from build123d import *

# Parameters (mm, degrees)
BOSS_EXTRUDE1_DEPTH = 1.6
FILLET1_R           = 5
SKETCH2_R           = 1.25
SKETCH2_W           = 17
SKETCH2_H           = 6.4
SKETCH2_W_2         = 30
SKETCH2_H_2         = 8
CUT_EXTRUDE1_DEPTH  = 3
FILLET2_R           = 2


with BuildPart() as part:
    # Sketch1 → Boss-Extrude1 (new body)
    with BuildSketch(Plane(origin=(0, 0, 0), x_dir=(1, 0, 0), z_dir=(0, 1, 0))):
        Polygon((-20, 55.916666667), (20, 55.916666667), (35, 30.916666667), (35, 25.916666667), (25, 25.916666667), (25, -22.083333333), (-25, -22.083333333), (-25, 25.916666667), (-35, 25.916666667), (-35, 30.916666667), align=None)
    extrude(amount=BOSS_EXTRUDE1_DEPTH)

    # Fillet1
    # the kernel refuses this fillet: 5 mm, written as the material it takes off along each edge
    with BuildSketch(Plane(origin=(-20, -7.077379737, -55.916666667), x_dir=(1, 0, 0), z_dir=(0, 1, 0))) as fillet1_piece_1:
        with BuildLine():
            CenterArc((FILLET1_R * 0.566190378969, -FILLET1_R), FILLET1_R, 90, 59.036243468)
            Line((-FILLET1_R * 0.291302546743, -FILLET1_R * 0.485504244572), (0, 0))
            Line((0, 0), (FILLET1_R * 0.566190378969, 0))
        make_face()
    extrude(amount=15.754759474, mode=Mode.SUBTRACT)
    with BuildSketch(Plane(origin=(20, -7.077379737, -55.916666667), x_dir=(-1, 0, 0), z_dir=(0, 1, 0))) as fillet1_piece_2:
        with BuildLine():
            CenterArc((FILLET1_R * 0.566190378969, FILLET1_R), FILLET1_R, 210.963756532, 59.036243468)
            Line((-FILLET1_R * 0.291302546743, FILLET1_R * 0.485504244572), (0, 0))
            Line((0, 0), (FILLET1_R * 0.566190378969, 0))
        make_face()
    extrude(amount=15.754759474, mode=Mode.SUBTRACT)
    with BuildSketch(Plane(origin=(-35, -3.462299562, -30.916666667), x_dir=(0, 0, 1), z_dir=(0, 1, 0)), Plane(origin=(35, -3.462299562, -30.916666667), x_dir=(-0.5144957554275258, 0, -0.8574929257125447), z_dir=(0, 1, 0))) as fillet1_piece_3:
        with BuildLine():
            CenterArc((FILLET1_R * 0.276983964948, FILLET1_R), FILLET1_R, 239.036243468, 30.963756532)
            Line((-FILLET1_R * 0.237511790479, FILLET1_R * 0.142507074287), (0, 0))
            Line((0, 0), (FILLET1_R * 0.276983964948, 0))
        make_face()
    extrude(amount=8.524599124, mode=Mode.SUBTRACT)
    with BuildSketch(Plane(origin=(-25, -12.5, 22.083333333), x_dir=(1, 0, 0), z_dir=(0, 1, 0)), Plane(origin=(25, -12.5, 22.083333333), x_dir=(0, 0, -1), z_dir=(0, 1, 0)), Plane(origin=(-35, -12.5, -25.916666667), x_dir=(1, 0, 0), z_dir=(0, 1, 0)), Plane(origin=(35, -12.5, -25.916666667), x_dir=(0, 0, -1), z_dir=(0, 1, 0))) as fillet1_piece_4:
        with BuildLine():
            CenterArc((FILLET1_R, FILLET1_R), FILLET1_R, 180, 90)
            Line((0, FILLET1_R), (0, 0))
            Line((0, 0), (FILLET1_R, 0))
        make_face()
    extrude(amount=26.6, mode=Mode.SUBTRACT)

    # Sketch2 → Cut-Extrude1 (cut)
    with BuildSketch(Plane(origin=(0, 0, 0), x_dir=(1, 0, 0), z_dir=(0, 1, 0))):
        with Locations(Location((22.5, -17.083333333, 0), (0, 0, 90))):
            Circle(SKETCH2_R)
        with Locations(Location((21.5, -4.403333333, 0), (0, 0, 90))):
            Circle(SKETCH2_R)
        with Locations(Location((17.9, 31.906666667, 0), (0, 0, 90))):
            Circle(SKETCH2_R)
        with Locations(Location((21.5, 12.226666667, 0), (0, 0, 90))):
            Circle(SKETCH2_R)
        with Locations(Location((-17.9, 31.906666667, 0), (0, 0, 90))):
            Circle(SKETCH2_R)
        with Locations(Location((-21.5, 12.226666667, 0), (0, 0, 90))):
            Circle(SKETCH2_R)
        with Locations(Location((-21.5, -4.403333333, 0), (0, 0, 90))):
            Circle(SKETCH2_R)
        with Locations(Location((-22.5, -17.083333333, 0), (0, 0, 90))):
            Circle(SKETCH2_R)
        with Locations((16.5, 3.896666667)):
            Rectangle(SKETCH2_W, SKETCH2_H)
        with Locations((-16.5, 3.896666667)):
            Rectangle(SKETCH2_W, SKETCH2_H)
        with Locations((0, 46.916666667)):
            Rectangle(SKETCH2_W_2, SKETCH2_H_2)
    extrude(amount=CUT_EXTRUDE1_DEPTH, mode=Mode.SUBTRACT)

    # Fillet2
    fillet2_edges = [part.edges().sort_by_distance(p)[0] for p in [
        (8, 0.8, -7.096666667),
        (8, 0.8, -0.696666667),
        (-8, 0.8, -0.696666667),
        (-8, 0.8, -7.096666667),
    ]]
    fillet(fillet2_edges, radius=FILLET2_R)


solid = part.part
Work out the finished part from the listing and answer in its coordinate system (mm). A direction names the side the tool comes from. Give positions to 0.01 mm unless a question says otherwise; leave off trailing zeros. Loops run counter-clockwise (first coordinate to the right, second up) from the corner with the lowest first, then second, coordinate; pieces in that order, holes last. Notation, with made-up numbers: (15.25, -1) - (23.25, -1) arc R21 ccw to (23.25, 31) - close; hole circle Ø6 at (85.5, 41). An arc over 180 degrees is marked (long way). Answer in a Markdown table with one row per item. Add a question column.
Q1. A tool of negligible diameter and unlimited length cuts with its end or side. For faces 1 (the cylindrical face through (8.57, 0.811, -6.495)), 2 (the flat face through (-18, 1, -0.697)), 3 (the flat face through (-27, 1, -25.917)), 4 (the flat face through (0, 1, -42.917)), from which of +Z, -Z, +X, -X, +Y, -Y can it reach the whole face along a straight path? Write none if from no direction.
Q2. The part is cut by section B-B (x = 11.5). Determine the outline of the cut face in (y, z), and give its area (3 significant figures).
Q3. Consider line 1 along Z through (x, y) = (-10, 1.3); line 2 along Z through (x, y) = (21.5, 0.6); line 3 along X through (y, z) = (1.5, -31.5). Determine where each line is inside the solid, lowest interval first.
Q4. Each of these flat-tipped pins is pushed along its axis until it touches: P1, Ø0.5, axis at y = 1, z = -4, coming from the -X side; P2, Ø0.8, axis at y = 0.5, z = 12, coming from the -X side; P3, Ø0.5, axis at y = 0.5, z = -16.5, coming from the +X side. Where does it stop, or does it pass through?
Q5. The part is cut by section A-A (x = -0.5). Determine the outline of the cut face in (y, z), and give its area (3 significant figures).
Q6. The part is cut by section C-C (y = 0.35). State how many separate pieces and enclosed holes the cut face has, and give its area (3 significant figures).
Q7. Determine the mould class of faces 5 (the cylindrical face through (-34.71, 0.79, -31.21)), 6 (the cylindrical face through (-20.28, 0.79, 4.67)), 7 (the flat face through (-25, 1, 8)) for opening direction Z: released by +Z, released by -Z, zero draft, split by the parting line, or undercut.
Solution:
| question | item | result |
|---|---|---|
| 1 | face 1 | +X, +Y, -Y |
| 1 | face 2 | -X, +Y, -Y |
| 1 | face 3 | +Z, -X, +Y, -Y |
| 1 | face 4 | +Y, -Y |
| 2 | outline | (0, -55.92) - (1.6, -55.92) - (1.6, -50.92) - (0, -50.92) - close; (0, -42.92) - (1.6, -42.92) - (1.6, -7.1) - (0, -7.1) - close; (0, -0.7) - (1.6, -0.7) - (1.6, 22.08) - (0, 22.08) - close |
| 2 | area | 102 mm² |
| 3 | line 1 | z = -55.92 to -50.92, -42.92 to -7.1, -0.7 to 22.08 |
| 3 | line 2 | z = -53.42 to -13.48, -10.98 to -7.1, -0.7 to 3.15, 5.65 to 16.33, 17.83 to 21.85 |
| 3 | line 3 | x = -34.6 to -19.08, -16.72 to 16.72, 19.08 to 34.6 |
| 4 | P1 | stops at x = -8 |
| 4 | P2 | stops at x = -25 |
| 4 | P3 | stops at x = 25 |
| 5 | outline | (0, -55.92) - (1.6, -55.92) - (1.6, -50.92) - (0, -50.92) - close; (0, -42.92) - (1.6, -42.92) - (1.6, 22.08) - (0, 22.08) - close |
| 5 | area | 112 mm² |
| 6 | separate pieces | 1 |
| 6 | enclosed holes | 9 |
| 6 | area | 3,610 mm² |
| 7 | face 5 | released by -Z |
| 7 | face 6 | undercut |
| 7 | face 7 | zero draft |
